from build123d import *

# Parameters (mm, degrees)
SKETCH_1_W          = 170
SKETCH_1_H          = 20
EXTRUDE_1_DEPTH     = 50
CUT_EXTRUDE_2_DEPTH = 164
SKETCH_3_R          = 5
CUT_EXTRUDE_3_DEPTH = 3
SKETCH_4_R          = 2.6
CUT_EXTRUDE_4_DEPTH = 3
SKETCH_5_W          = 170
SKETCH_5_H          = 20
CUT_EXTRUDE_5_DEPTH = 400
SKETCH_6_R          = 5
CUT_EXTRUDE_6_DEPTH = 400
SKETCH_7_R          = 5
SKETCH_7_R_2        = 2.6
EXTRUDE_2_DEPTH     = 3
SKETCH_8_W          = 35
SKETCH_8_H          = 3.05
SKETCH_8_W_2        = 80
EXTRUDE_3_DEPTH     = 4
SKETCH_9_W          = 6.1
SKETCH_9_H          = 30
EXTRUDE_4_DEPTH     = 4


with BuildPart() as part:
    # 草图1 → 凸台-拉伸1 (new body)
    with BuildSketch(Plane(origin=(0, 0, 0), x_dir=(1, 0, 0), z_dir=(0, 1, 0))):
        with Locations((85, 10)):
            Rectangle(SKETCH_1_W, SKETCH_1_H)
    extrude_1 = extrude(amount=EXTRUDE_1_DEPTH)

    # 草图2 → 切除-拉伸2 (cut)
    with BuildSketch(Plane(origin=(170, 0, 0), x_dir=(0, 0, -1), z_dir=(1, 0, 0))):
        Polygon((0, 50), (20, 0), (20, 50), align=None)
    cut_extrude_2 = extrude(amount=-CUT_EXTRUDE_2_DEPTH, mode=Mode.SUBTRACT)

    # 草图3 → 切除-拉伸3 (cut)
    with BuildSketch(Plane(origin=(6, 0, 0), x_dir=(0, 0, -1), z_dir=(1, 0, 0))):
        with Locations((10, 40)):
            Circle(SKETCH_3_R)
    cut_extrude_3 = extrude(amount=-CUT_EXTRUDE_3_DEPTH, mode=Mode.SUBTRACT)

    # 草图4 → 切除-拉伸4 (cut)
    with BuildSketch(Plane(origin=(3, 0, 0), x_dir=(0, 0, -1), z_dir=(1, 0, 0))):
        with Locations((10, 40)):
            Circle(SKETCH_4_R)
    cut_extrude_4 = extrude(amount=-CUT_EXTRUDE_4_DEPTH, mode=Mode.SUBTRACT)

    # 镜向1: 凸台-拉伸1, 切除-拉伸2, 切除-拉伸3, 切除-拉伸4 across plane
    add(extrude_1.mirror(Plane(origin=(170, 50, 0), x_dir=(0, 0, 1), z_dir=(-1, 0, 0))))
    add(cut_extrude_2.mirror(Plane(origin=(170, 50, 0), x_dir=(0, 0, 1), z_dir=(-1, 0, 0))), mode=Mode.SUBTRACT)
    add(cut_extrude_3.mirror(Plane(origin=(170, 50, 0), x_dir=(0, 0, 1), z_dir=(-1, 0, 0))), mode=Mode.SUBTRACT)
    add(cut_extrude_4.mirror(Plane(origin=(170, 50, 0), x_dir=(0, 0, 1), z_dir=(-1, 0, 0))), mode=Mode.SUBTRACT)

    # 草图5 → 切除-拉伸5 (cut)
    with BuildSketch(Plane.XZ):
        with Locations((85, -10)):
            Rectangle(SKETCH_5_W, SKETCH_5_H)
    extrude(amount=-CUT_EXTRUDE_5_DEPTH, mode=Mode.SUBTRACT)

    # 草图6 → 切除-拉伸6 (cut)
    with BuildSketch(Plane.XZ):
        with Locations(Location((231.37, -10, 0), (0, 0, 270))):
            Circle(SKETCH_6_R)
    extrude(amount=-CUT_EXTRUDE_6_DEPTH, mode=Mode.SUBTRACT)

    # 草图7 → 凸台-拉伸2 (add)
    with BuildSketch(Plane.XZ):
        with Locations(Location((231.37, -10, 0), (0, 0, 270))):
            Circle(SKETCH_7_R)
        with Locations(Location((231.37, -10, 0), (0, 0, 270))):
            Circle(SKETCH_7_R_2, mode=Mode.SUBTRACT)
    extrude(amount=-EXTRUDE_2_DEPTH)

    # 草图8 → 凸台-拉伸3 (add)
    with BuildSketch(Plane.XZ):
        with Locations((187.5, -8.475)):
            Rectangle(SKETCH_8_W, SKETCH_8_H)
        with Locations((187.5, -11.525)):
            Rectangle(SKETCH_8_W, SKETCH_8_H)
        with Locations((300, -8.475)):
            Rectangle(SKETCH_8_W_2, SKETCH_8_H)
        with Locations((300, -11.525)):
            Rectangle(SKETCH_8_W_2, SKETCH_8_H)
    extrude(amount=EXTRUDE_3_DEPTH)

    # 草图9 → 凸台-拉伸4 (add)
    with BuildSketch(Plane(origin=(340, 0, 0), x_dir=(0, 0, -1), z_dir=(1, 0, 0))):
        with Locations((10, 15)):
            Rectangle(SKETCH_9_W, SKETCH_9_H)
    extrude(amount=EXTRUDE_4_DEPTH)


solid = part.part
Source: CAD feature listing. Evaluate the final solid. Frame: model axes, mm. A direction names the side the tool comes from. Give positions to 0.01 mm unless a question says otherwise; leave off trailing zeros. Loops run counter-clockwise (first coordinate to the right, second up) from the corner with the lowest first, then second, coordinate; pieces in that order, holes last. Notation, with made-up numbers: (85.5, -1) -> (97.5, -1) arc R19 ccw to (97.5, 32) -> close; hole circle Ø9 at (87.5, 31.25). An arc over 180 degrees is marked (long way). Use a Markdown table: item, result. Add a question column.
1) Section query D-D, the plane y = 6.5. Return the cut outline in (x, z), then the cut area to 3 significant figures.
2) Pull-direction query (Z, two-part tool) for faces 1 (the face through (187, -4, -10)), 2 (the face through (231.59, 16.373, -5.005)), 3 (the face through (256, 25, 0)), 4 (the face through (337, 38, -12)); classes: +Z half, -Z half, draft (parallel to the pull), parting line (faces both ways), or undercut.
3) Section query A-A, the plane z = -10. Count the separate pieces of the cut face and the enclosed holes in it, then the cut area to 3 significant figures.
4) Reachability of faces 5 (the face through (342, 15, -6.95)), 6 (the face through (187, -2, -6.95)), 7 (the face through (187, -2, -13.05)), 8 (the face through (342, 0, -10)), 9 (the face through (334, 31, -14)) from +Z, -Z, +X, -X, +Y, -Y: full face, straight path, thin tool, end or side. Return the list, or none.
5) Section query B-B, the plane y = 40. Return the cut outline in (x, z), then the cut area to 3 significant figures.
6) Line query: line 1 along Y through (x, z) = (335.2, -10); line 2 along X through (y, z) = (28.5, -15.75); line 3 along Y through (x, z) = (339.35, -10). Output: solid intervals per line, ascending. Write a range as [from, to].
7) Section query C-C, the plane x = 231.37. Return the cut outline in (y, z), then the cut area to 3 significant figures.
8) First-contact query: pin 1 (3 mm diameter, centred on x = 343, y = 21, fed in from -Z); pin 2 (10 mm diameter, centred on x = 263, z = -13.5, fed in from -Y); pin 3 (3 mm diameter, centred on x = 295.5, y = -2, fed in from +Z); pin 4 (1.2 mm diameter, centred on x = 342.5, y = 21, fed in from +Z). Flat tips, straight axial feed; report the tip coordinate or a pass-through.
Numbers:
| question | item | result |
|---|---|---|
| 1 | outline | (170, -17.4) -> (334, -17.4) -> (334, -20) -> (340, -20) -> (340, -13.05) -> (344, -13.05) -> (344, -6.95) -> (340, -6.95) -> (340, 0) -> (170, 0) -> close; hole circle Ø10 at (231.37, -10) |
| 1 | area | 2,920 mm2 |
| 2 | face 1 | draft |
| 2 | face 2 | undercut |
| 2 | face 3 | +Z half |
| 2 | face 4 | undercut |
| 3 | separate pieces | 3 |
| 3 | enclosed holes | 0 |
| 3 | area | 4,700 mm2 |
| 4 | face 5 | +Z, +X, +Y, -Y |
| 4 | face 6 | +Z, +X, -X, -Y |
| 4 | face 7 | -Z, +X, -X, -Y |
| 4 | face 8 | +Z, -Z, +X, -Y |
| 4 | face 9 | -Z, -X, +Y |
| 5 | outline | (170, -4) -> (334, -4) -> (334, -5) -> (337, -5) -> (337, -7.4) -> (340, -7.4) -> (340, 0) -> (170, 0) -> close; (334, -20) -> (340, -20) -> (340, -12.6) -> (337, -12.6) -> (337, -15) -> (334, -15) -> close |
| 5 | area | 730 mm2 |
| 6 | line 1 | y = [-4, 35], [45, 50] |
| 6 | line 2 | x = [334, 340] |
| 6 | line 3 | y = [-4, 37.4], [42.6, 50] |
| 7 | outline | (0, -20) -> (12.5, -15) -> (3, -15) -> (3, -12.6) -> (0, -12.6) -> close; (0, -7.4) -> (3, -7.4) -> (3, -5) -> (37.5, -5) -> (50, 0) -> (0, 0) -> close |
| 7 | area | 264 mm2 |
| 8 | pin 1 | stops at z = -13.05 |
| 8 | pin 2 | stops at y = -4 |
| 8 | pin 3 | stops at z = -6.95 |
| 8 | pin 4 | stops at z = -6.95 |
